The model under review builds one solid part; all positions refer to its coordinate system, in mm. Face numbers are marked on the shaded views. A direction names the side the tool comes from. Coordinates: 2 decimals unless noted, no trailing zeros. Write each loop counter-clockwise with the first axis right and the second up, starting at its lowest first coordinate (ties: lowest second). Pieces come first, ordered by that corner, then holes.
1) Add section C-C, the plane z = 1.5. State the section outline as (x, y) points.
2) For P1, Ø3, axis at x = 0.5, y = 9.5, coming from the -Z side; P2, Ø2, axis at y = 2.5, z = 5.5, coming from the -X side, all flat-tipped, find the tip position at first contact; note any pin that passes through.
3) Machinability: for the marked faces 1 and 2, which of the approach directions +Z, -Z, +X, -X, +Y, -Y give a long, thin tool a straight path to every point of the face, cutting with its end or side? Answer none if there is none.
4) Add section D-D, the plane z = 5. State the section outline as (x, y) points, then the cut area to 3 significant figures.
5) Add section A-A, the plane y = 0. State the section outline as (x, z) points.
6) For line 1 (Y direction, x = 0, z = 5.55); line 2 (X direction, y = -1.75, z = 5.5); line 3 (X direction, y = 2, z = 0.5), list the stretches that pass through material, from the lowest coordinate up.
7) Mouldability with a two-part tool opening along X and no side actions: class the marked faces 3, 4 and 5 as released by +X, released by -X, zero draft, split by the parting line, or undercut.
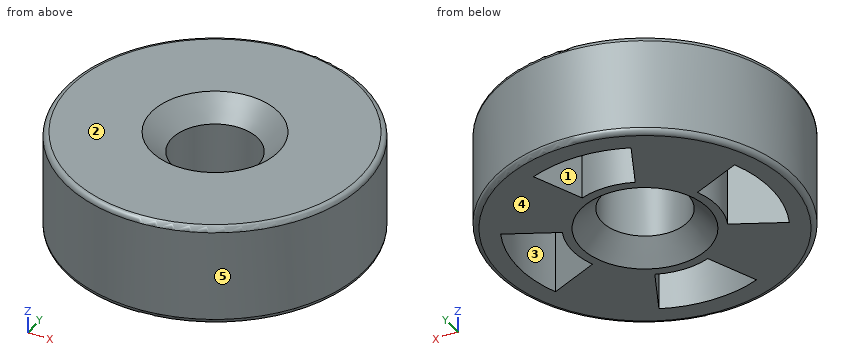
from build123d import *

# Parameters (mm, degrees)
F0_R     = 14.5
F0_R_2   = 4.15
F1_DEPTH = 9.8
F2_SIZE  = 2
F4_DEPTH = 7.8
F5_R     = 0.5


with BuildPart() as f1:
    # F0 (on Top) → F1 (new body)
    with BuildSketch(Plane.XY):
        Circle(F0_R)
        Circle(F0_R_2, mode=Mode.SUBTRACT)
    extrude(amount=F1_DEPTH)

    # F2
    f2_edges = [f1.edges().sort_by_distance(p)[0] for p in [
        (-4.15, 0, 9.8),
        (-4.15, 0, 0),
    ]]
    chamfer(f2_edges, length=F2_SIZE)

    # F3 (on face) → F4 (cut)
    with BuildSketch(Plane(origin=(0, 0, 0), x_dir=(1, 0, 0), z_dir=(0, 0, -1))):
        with BuildLine():
            Line((2.53053, 6.526593), (4.653059, 11.277812))
            ThreePointArc((4.653059, 11.277812), (0, 12.2), (-4.653059, 11.277812))
            Line((-4.653059, 11.277812), (-2.53053, 6.526593))
            ThreePointArc((-2.53053, 6.526593), (0, 7), (2.53053, 6.526593))
        make_face()
        with BuildLine():
            Line((-6.453522, 2.711468), (-11.163082, 4.92195))
            ThreePointArc((-11.163082, 4.92195), (-12.2, 0), (-11.163082, -4.92195))
            Line((-11.163082, -4.92195), (-6.453522, -2.711468))
            ThreePointArc((-6.453522, -2.711468), (-7, 0), (-6.453522, 2.711468))
        make_face()
        with BuildLine():
            Line((4.653059, -11.277812), (2.53053, -6.526593))
            ThreePointArc((2.53053, -6.526593), (0, -7), (-2.53053, -6.526593))
            Line((-2.53053, -6.526593), (-4.653059, -11.277812))
            ThreePointArc((-4.653059, -11.277812), (0, -12.2), (4.653059, -11.277812))
        make_face()
        with BuildLine():
            Line((11.163082, 4.92195), (6.453522, 2.711468))
            ThreePointArc((6.453522, 2.711468), (7, 0), (6.453522, -2.711468))
            Line((6.453522, -2.711468), (11.163082, -4.92195))
            ThreePointArc((11.163082, -4.92195), (12.2, 0), (11.163082, 4.92195))
        make_face()
    extrude(amount=-F4_DEPTH, mode=Mode.SUBTRACT)

    # F5
    f5_edges = [f1.edges().sort_by_distance(p)[0] for p in [
        (-14.5, 0, 9.8),
        (-14.5, 0, 0),
    ]]
    fillet(f5_edges, radius=F5_R)


solid = f1.part
Geometry results:
1. outline: circle Ø29 at (0, 0); hole (-11.16, -4.92) - (-6.45, -2.71) arc R7 cw to (-6.45, 2.71) - (-11.16, 4.92) arc R12.2 ccw to start; hole (-4.65, -11.28) arc R12.2 ccw to (4.65, -11.28) - (2.53, -6.53) arc R7 cw to (-2.53, -6.53) - close; hole circle Ø9.3 at (0, 0); hole (-4.65, 11.28) - (-2.53, 6.53) arc R7 cw to (2.53, 6.53) - (4.65, 11.28) arc R12.2 ccw to start; hole (6.45, -2.71) - (11.16, -4.92) arc R12.2 ccw to (11.16, 4.92) - (6.45, 2.71) arc R7 cw to start
2. P1: stops at z = 7.8
2. P2: stops at x = -14.42
3. face 1: -Z
3. face 2: +Z, +X, -X, +Y, -Y
4. outline: circle Ø29 at (0, 0); hole (-11.16, -4.92) - (-6.45, -2.71) arc R7 cw to (-6.45, 2.71) - (-11.16, 4.92) arc R12.2 ccw to start; hole (-4.65, -11.28) arc R12.2 ccw to (4.65, -11.28) - (2.53, -6.53) arc R7 cw to (-2.53, -6.53) - close; hole (-4.65, 11.28) - (-2.53, 6.53) arc R7 cw to (2.53, 6.53) - (4.65, 11.28) arc R12.2 ccw to start; hole circle Ø8.3 at (0, 0); hole (6.45, -2.71) - (11.16, -4.92) arc R12.2 ccw to (11.16, 4.92) - (6.45, 2.71) arc R7 cw to start
4. area: 448 mm2
5. outline: (-14.5, 0.5) arc R0.5 ccw to (-14, 0) - (-12.2, 0) - (-12.2, 7.8) - (-7, 7.8) - (-7, 0) - (-6.15, 0) - (-4.15, 2) - (-4.15, 7.8) - (-6.15, 9.8) - (-14, 9.8) arc R0.5 ccw to (-14.5, 9.3) - close; (4.15, 2) - (6.15, 0) - (7, 0) - (7, 7.8) - (12.2, 7.8) - (12.2, 0) - (14, 0) arc R0.5 ccw to (14.5, 0.5) - (14.5, 9.3) arc R0.5 ccw to (14, 9.8) - (6.15, 9.8) - (4.15, 7.8) - close
6. line 1: y = -14.5 to -12.2, -7 to -4.15, 4.15 to 7, 12.2 to 14.5
6. line 2: x = -14.39 to -12.07, -6.78 to -3.76, 3.76 to 6.78, 12.07 to 14.39
6. line 3: x = -14.36 to -12.03, -6.71 to -5.28, 5.28 to 6.71, 12.03 to 14.36
7. face 3: undercut
7. face 4: zero draft
7. face 5: split by the parting line
